Source: CAD feature listing. Evaluate the final solid. Frame: model axes, mm. A direction names the side the tool comes from. Coordinates: 2 decimals unless noted, no trailing zeros. Loops run counter-clockwise (first coordinate to the right, second up) from the corner with the lowest first, then second, coordinate; pieces in that order, holes last. Notation, with made-up numbers: (-7.75, -38) -> (-2.75, -38) arc R37 cw to (-2.75, -1) -> close; hole circle Ø7 at (9.5, 43). An arc over 180 degrees is marked (long way). Answer as CSV lines item,"result".
from build123d import *

# Parameters (mm, degrees)
F0_R     = 4.7625
F1_DEPTH = 6.35
F2_DEPTH = 101.6


with BuildPart() as f1:
    # F0 (on Right) → F1 (new body)
    with BuildSketch(Plane.YZ):
        Polygon((7.14375, -4.124446), (7.14375, 4.124446), (0, 8.248892), (-7.14375, 4.124446), (-7.14375, -4.124446), (0, -8.248892), align=None)
        Circle(F0_R, mode=Mode.SUBTRACT)
        Circle(F0_R)
    extrude(amount=-F1_DEPTH)

    # F0 (on Right) → F2 (join)
    with BuildSketch(Plane.YZ):
        Circle(F0_R)
    extrude(amount=F2_DEPTH)


solid = f1.part
(1) Cut plane A-A (z = 0). Return the cut outline in (x, y).
Computed values:
outline,"(-6.35, -7.14) -> (0, -7.14) -> (0, -4.76) -> (101.6, -4.76) -> (101.6, 4.76) -> (0, 4.76) -> (0, 7.14) -> (-6.35, 7.14) -> close"
(2) Pin query (flat end, axial travel): pin 1 Ø4 at (x, y) = (60, 3.5) entering from -Z; pin 2 Ø2 at (x, y) = (6.5, -4) entering from -Z; pin 3 Ø8 at (x, y) = (45, 3.5) entering from +Z. Return the tip coordinate at first contact, or that it passes through.
Computed values:
pin 1,"z = -4.52"
pin 2,"z = -3.7"
pin 3,"z = 4.76"
(3) Cut plane D-D (z = -6.5). Return the cut outline in (x, y).
Computed values:
outline,"(-6.35, -3.03) -> (0, -3.03) -> (0, 3.03) -> (-6.35, 3.03) -> close"
(4) Access query for faces 5 (the flat face through (0, -3, -4)), 6 (the flat face through (-3.131, 3.522, -6.216)). Directions: +Z, -Z, +X, -X, +Y, -Y. A direction counts if a zero-diameter tool reaches every point of the face in a straight line with its end or side. Return the directions, or none.
Computed values:
face 5,"+X"
face 6,"-Z, +X, -X, +Y"
(5) Material intervals for L1, parallel to X at y = -5.5, z = 0; L2, parallel to Y at x = 75, z = -0.25; L3, parallel to Z at x = 48, y = -4.25, sorted ascending. Write a range as [from, to].
Computed values:
L1,"[-6.35, 0]"
L2,"[-4.76, 4.76]"
L3,"[-2.15, 2.15]"
(6) Cut plane C-C (x = 88). Return the cut outline in (y, z) (1 decimal), then the cut area to 3 significant figures.
Computed values:
outline,"circle Ø9.5 at (0, 0)"
area,"71.3 mm^2"
(7) Cut plane B-B (y = -2). Return the cut outline in (x, z), then the cut area to 3 significant figures.
Computed values:
outline,"(-6.35, -7.09) -> (0, -7.09) -> (0, -4.32) -> (101.6, -4.32) -> (101.6, 4.32) -> (0, 4.32) -> (0, 7.09) -> (-6.35, 7.09) -> close"
area,"968 mm^2"
(8) Draft query along Y for faces 1 (the cylindrical face through (50.09, -3.78, -2.9)), 2 (the flat face through (-3, -7.144, 0)), 3 (the flat face through (-3.13, 3.62, 6.16)), 4 (the flat face through (101.6, 0, 0)). Return one class per face: released by +Y, released by -Y, zero draft, split by the parting line, or undercut.
Computed values:
face 1,"split by the parting line"
face 2,"released by -Y"
face 3,"released by +Y"
face 4,"zero draft"
